Part model, mm, in its own coordinate system. Face numbers are marked on the shaded views. A direction names the side the tool comes from. Round coordinates to 2 decimals unless told otherwise and drop trailing zeros. Write each loop counter-clockwise with the first axis right and the second up, starting at its lowest first coordinate (ties: lowest second). Pieces come first, ordered by that corner, then holes. Notation, with made-up numbers: (62, -9) -> (80, -9) arc R7 ccw to (80, -5) -> close; hole circle Ø4 at (-13, 80.25). An arc over 180 degrees is marked (long way). Use CSV: the item, a comma, the result in double quotes. Start each with the question number.
(1) Two-plate mould, pull along X, no slides. Class the marked faces 1, 2 and 3: released by +X, released by -X, zero draft, split by the parting line, or undercut.
(2) Drop flat-ended pins along their axis: pin 1 (2 mm diameter, centred on x = 18.5, z = 3, fed in from +Y); pin 2 (2 mm diameter, centred on x = 18, z = 2.5, fed in from -Y); pin 3 (0.5 mm diameter, centred on y = -0.5, z = 4.5, fed in from +X). Give the stop position or say it passes through.
(3) Probe line 1 (Y direction, x = 17.25, z = 0.65); line 2 (Y direction, x = 21.5, z = 3.9); line 3 (X direction, y = 1.75, z = 0.35). List the from-to ranges inside material, lowest first. Write a range as [from, to].
(4) Saw through at A-A (x = 21). Give the cut face in (y, z).
(5) Which spindle directions (+Z, -Z, +X, -X, +Y, -Y) get a long thin tool onto all of the face, cutting with end or side? Do the marked faces 4, 5, 6 and 7. Say none if no direction does.
(6) Saw through at B-B (y = 3). Give the cut face in (x, z), plus the area to 3 significant figures.
(7) Saw through at C-C (y = 5.5). Give the cut face in (x, z).
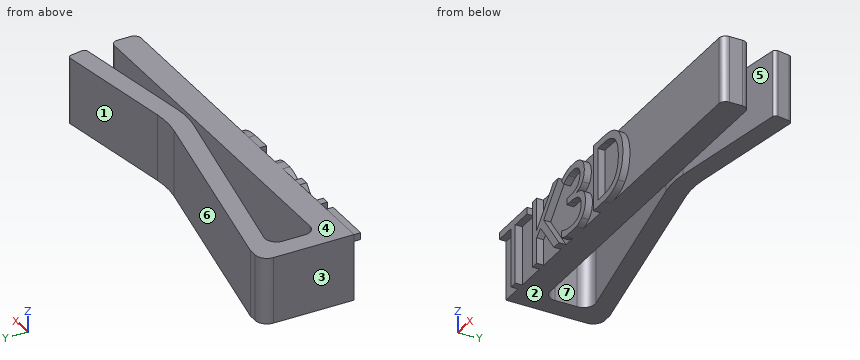
```python
from build123d import *

# Parameters (mm, degrees)
F1_DEPTH = 4.826
F2_R     = 0.8421318362
F3_R     = 0.8368220374
F4_R     = 0.4905681959
F5_R     = 0.7971733183
F7_DEPTH = 0.508
F8_R     = 0.4905681959


with BuildPart() as f1:
    # F0 (on Top) → F1 (new body)
    with BuildSketch(Plane.XY):
        Polygon((3.7636798806, 1.93111517), (3.7636798806, 0), (31.9592878222, 0), (31.9592878222, 1.93111517), (5.2430788055, 1.93111517), align=None)
        with BuildLine():
            Line((3.7636798806, 6.3693127595), (3.7636798806, 1.93111517))
            Line((3.7636798806, 1.93111517), (5.2430788055, 1.93111517))
            Line((5.2430788055, 1.93111517), (5.2430788055, 5.3456245812))
            Line((5.2430788055, 5.3456245812), (20.4440524117, 2.3154419081))
            ThreePointArc((20.4440524117, 2.3154419081), (21.572559685, 2.1939202222), (22.7046736444, 2.2752477642))
            Line((22.7046736444, 2.2752477642), (31.7002432299, 3.7380780613))
            ThreePointArc((31.7002432299, 3.7380780613), (31.8710772939, 3.8437373318), (31.9171628323, 4.0392476436))
            Line((31.9171628323, 4.0392476436), (31.7757464521, 4.9088774915))
            ThreePointArc((31.7757464521, 4.9088774915), (31.6700871816, 5.0797115555), (31.4745768698, 5.1257970939))
            Line((31.4745768698, 5.1257970939), (22.6872542576, 3.696831243))
            ThreePointArc((22.6872542576, 3.696831243), (21.5722351198, 3.6152227731), (20.4601853424, 3.7304309004))
            Line((20.4601853424, 3.7304309004), (5.2430788055, 6.6787209362))
            Line((5.2430788055, 6.6787209362), (3.7601878867, 6.6787209362))
            Line((3.7601878867, 6.6787209362), (3.7636798806, 6.3693127595))
        make_face()
    extrude(amount=F1_DEPTH)

    # F2
    f2_edges = [f1.edges().sort_by_distance(p)[0] for p in [
        (3.760188, 6.678721, 2.413),
    ]]
    fillet(f2_edges, radius=F2_R)

    # F3
    f3_edges = [f1.edges().sort_by_distance(p)[0] for p in [
        (5.243079, 5.345625, 2.413),
    ]]
    fillet(f3_edges, radius=F3_R)

    # F4
    f4_edges = [f1.edges().sort_by_distance(p)[0] for p in [
        (31.959288, 1.931115, 2.413),
    ]]
    fillet(f4_edges, radius=F4_R)

    # F5
    f5_edges = [f1.edges().sort_by_distance(p)[0] for p in [
        (5.243079, 1.931115, 2.413),
    ]]
    fillet(f5_edges, radius=F5_R)

    # F6 (on face) → F7 (join)
    with BuildSketch(Plane.XZ):
        Polygon((5.3377853494, 0), (5.8939064431, 0), (5.8939064431, 4.2908250868), (7.4093626063, 4.2908250868), (7.4093626063, 4.7851549479), (3.8223291862, 4.7851549479), (3.8223291862, 4.2908250868), (5.3377853494, 4.2908250868), align=None)
        Polygon((8.1299112175, 4.7851549479), (8.1299112175, 0), (8.6860323112, 0), (8.6860323112, 1.8757304688), (9.1876933355, 2.3208368056), (10.9314628668, 0), (11.5860310091, 0), (9.5898600022, 2.7062465278), (11.5137666862, 4.7851549479), (10.8560566168, 4.7851549479), (8.6860323112, 2.411952691), (8.6860323112, 4.7851549479), align=None)
        with BuildLine():
            Line((13.789949635, 4.826), (13.0315141767, 4.826))
            add(Edge.make_bspline(
                [(12.598778839, 4.7207454427), (12.8088874261, 4.7931670674), (13.0315141767, 4.826)],
                knots=[0, 0, 0, 0.5466418669, 0.5466418669, 0.5466418669], degree=2))
            add(Edge.make_bspline(
                [(11.920122589, 4.3557582465), (12.2144164258, 4.5882608507), (12.598778839, 4.7207454427)],
                knots=[0, 0, 0, 1, 1, 1], degree=2))
            Line((11.920122589, 4.3557582465), (12.1945175543, 3.9892000868))
            add(Edge.make_bspline(
                [(12.8297104796, 4.3039164497), (12.5516499327, 4.2185607639), (12.1945175543, 3.9892000868)],
                knots=[0, 0, 0, 1, 1, 1], degree=2))
            add(Edge.make_bspline(
                [(13.4219637348, 4.3892721354), (13.1077710265, 4.3892721354), (12.8297104796, 4.3039164497)],
                knots=[0, 0, 0, 1, 1, 1], degree=2))
            add(Edge.make_bspline(
                [(14.0749609136, 4.1892361111), (13.8346034918, 4.3892721354), (13.4219637348, 4.3892721354)],
                knots=[0, 0, 0, 1, 1, 1], degree=2))
            add(Edge.make_bspline(
                [(14.3153183355, 3.6393988715), (14.3153183355, 3.9892000868), (14.0749609136, 4.1892361111)],
                knots=[0, 0, 0, 1, 1, 1], degree=2))
            add(Edge.make_bspline(
                [(13.9880342643, 2.9534114583), (14.3153183355, 3.2005763889), (14.3153183355, 3.6393988715)],
                knots=[0, 0, 0, 1, 1, 1], degree=2))
            add(Edge.make_bspline(
                [(13.1014871723, 2.7062465278), (13.6607501931, 2.7062465278), (13.9880342643, 2.9534114583)],
                knots=[0, 0, 0, 1, 1, 1], degree=2))
            Line((13.1014871723, 2.7062465278), (12.6239142556, 2.7062465278))
            Line((12.6239142556, 2.7062465278), (12.6239142556, 2.2391467014))
            Line((12.6239142556, 2.2391467014), (13.0952033181, 2.2391467014))
            add(Edge.make_bspline(
                [(14.4629889084, 1.3677855903), (14.4629889084, 2.2391467014), (13.0952033181, 2.2391467014)],
                knots=[0, 0, 0, 1, 1, 1], degree=2))
            add(Edge.make_bspline(
                [(13.2229750195, 0.3958828125), (14.4629889084, 0.3958828125), (14.4629889084, 1.3677855903)],
                knots=[0, 0, 0, 1, 1, 1], degree=2))
            add(Edge.make_bspline(
                [(12.5568864779, 0.4760019531), (12.9087823112, 0.3958828125), (13.2229750195, 0.3958828125)],
                knots=[0, 0, 0, 1, 1, 1], degree=2))
            add(Edge.make_bspline(
                [(11.8939398633, 0.7100755208), (12.2049906445, 0.5561210938), (12.5568864779, 0.4760019531)],
                knots=[0, 0, 0, 1, 1, 1], degree=2))
            Line((11.8939398633, 0.7100755208), (11.8939398633, 0.1927048611))
            add(Edge.make_bspline(
                [(12.4635495715, 0), (12.1708045154, 0.0591469127), (11.8939398633, 0.1927048611)],
                knots=[0.0691615274, 0.0691615274, 0.0691615274, 1, 1, 1], degree=2))
            Line((12.4635495715, 0), (13.8707030072, 0))
            add(Edge.make_bspline(
                [(14.5509628668, 0.302672309), (14.277243255, 0.0899806901), (13.8707030072, 0)],
                knots=[0, 0, 0, 0.5769429439, 0.5769429439, 0.5769429439], degree=2))
            add(Edge.make_bspline(
                [(15.0253938563, 1.3552178819), (15.0253938563, 0.6713250868), (14.5509628668, 0.302672309)],
                knots=[0, 0, 0, 1, 1, 1], degree=2))
            add(Edge.make_bspline(
                [(14.7473333095, 2.1276082899), (15.0253938563, 1.8327907986), (15.0253938563, 1.3552178819)],
                knots=[0, 0, 0, 1, 1, 1], degree=2))
            add(Edge.make_bspline(
                [(13.8932527973, 2.4936427951), (14.4692727626, 2.4224257813), (14.7473333095, 2.1276082899)],
                knots=[0, 0, 0, 1, 1, 1], degree=2))
            Line((13.8932527973, 2.4936427951), (13.8932527973, 2.5198255208))
            add(Edge.make_bspline(
                [(14.6216562261, 2.9094244792), (14.3645418598, 2.6182725694), (13.8932527973, 2.5198255208)],
                knots=[0, 0, 0, 1, 1, 1], degree=2))
            add(Edge.make_bspline(
                [(14.8787705925, 3.6592977431), (14.8787705925, 3.2005763889), (14.6216562261, 2.9094244792)],
                knots=[0, 0, 0, 1, 1, 1], degree=2))
            add(Edge.make_bspline(
                [(14.4923135612, 4.5343244358), (14.8787705925, 4.2154188368), (14.8787705925, 3.6592977431)],
                knots=[0, 0, 0, 1, 1, 1], degree=2))
            add(Edge.make_bspline(
                [(13.789949635, 4.826), (14.2187826063, 4.7600430693), (14.4923135612, 4.5343244358)],
                knots=[0.2922086215, 0.2922086215, 0.2922086215, 1, 1, 1], degree=2))
        make_face()
        with BuildLine():
            Line((16.0758448112, 4.7851549479), (16.0758448112, 0))
            Line((16.0758448112, 0), (17.4017380404, 0))
            add(Edge.make_bspline(
                [(19.2523330925, 0.6268144531), (18.6092853494, 0), (17.4017380404, 0)],
                knots=[0, 0, 0, 1, 1, 1], degree=2))
            add(Edge.make_bspline(
                [(19.8953808355, 2.4381354167), (19.8953808355, 1.2536289063), (19.2523330925, 0.6268144531)],
                knots=[0, 0, 0, 1, 1, 1], degree=2))
            add(Edge.make_bspline(
                [(19.2769448546, 4.166718967), (19.8953808355, 3.5482829861), (19.8953808355, 2.4381354167)],
                knots=[0, 0, 0, 1, 1, 1], degree=2))
            add(Edge.make_bspline(
                [(17.5420774501, 4.7851549479), (18.6585088737, 4.7851549479), (19.2769448546, 4.166718967)],
                knots=[0, 0, 0, 1, 1, 1], degree=2))
            Line((17.5420774501, 4.7851549479), (16.0758448112, 4.7851549479))
        make_face()
        with BuildLine():
            add(Edge.make_bspline(
                [(19.3067931619, 2.4182365451), (19.3067931619, 3.354530816), (18.8370750629, 3.8289618056)],
                knots=[0, 0, 0, 1, 1, 1], degree=2))
            add(Edge.make_bspline(
                [(18.8056557921, 0.9703318142), (19.3067931619, 1.4599487847), (19.3067931619, 2.4182365451)],
                knots=[0, 0, 0, 1, 1, 1], degree=2))
            add(Edge.make_bspline(
                [(17.3095748459, 0.4807148438), (18.3045184223, 0.4807148438), (18.8056557921, 0.9703318142)],
                knots=[0, 0, 0, 1, 1, 1], degree=2))
            Line((17.3095748459, 0.4807148438), (16.631965905, 0.4807148438))
            Line((16.631965905, 0.4807148437), (16.631965905, 4.3033927951))
            Line((16.631965905, 4.3033927951), (17.4404884744, 4.3033927951))
            add(Edge.make_bspline(
                [(18.8370750629, 3.8289618056), (18.367356964, 4.3033927951), (17.4404884744, 4.3033927951)],
                knots=[0, 0, 0, 1, 1, 1], degree=2))
        make_face(mode=Mode.SUBTRACT)
    extrude(amount=F7_DEPTH)

    # F8
    f8_edges = [f1.edges().sort_by_distance(p)[0] for p in [
        (31.959288, 0, 2.413),
    ]]
    fillet(f8_edges, radius=F8_R)


solid = f1.part
```
Answers:
1,face 1,"undercut"
1,face 2,"zero draft"
1,face 3,"released by -X"
2,pin 1,"stops at y = 4.3"
2,pin 2,"stops at y = 0"
2,pin 3,"stops at x = 19.19"
3,line 1,"y = [0, 1.93], [2.95, 4.35]"
3,line 2,"y = [0, 1.93], [2.2, 3.62]"
3,line 3,"x = [3.76, 31.85]"
4,outline,"(0, 0) -> (1.93, 0) -> (1.93, 4.83) -> (0, 4.83) -> close; (2.23, 0) -> (3.65, 0) -> (3.65, 4.83) -> (2.23, 4.83) -> close"
5,face 4,"+Z, +X, -X, +Y, -Y"
5,face 5,"+Z, -Z, +X"
5,face 6,"+Z, -Z, +Y"
5,face 7,"+Z, -Z"
6,outline,"(3.76, 0) -> (5.24, 0) -> (5.24, 4.83) -> (3.76, 4.83) -> close; (17.01, 0) -> (27.16, 0) -> (27.16, 4.83) -> (17.01, 4.83) -> close"
6,area,"56.1 mm²"
7,outline,"(3.76, 0) -> (11.33, 0) -> (11.33, 4.83) -> (3.76, 4.83) -> close"
